Could you check a few things on this drawing? It's one solid part, dimensions in mm from its lowest x, y, z. Coordinates: 2 decimals unless noted, no trailing zeros. Order: outer loops, then holes, each group sorted by start corner. A loop starts at its lowest first (then second) coordinate and runs counter-clockwise, first axis right, second up. Notation, with made-up numbers: (31.25, 37.25) - (73.25, 37.25) arc R19 ccw to (73.25, 60.25) - close; hole circle Ø2 at (62, 21.25). An arc over 180 degrees is marked (long way). Answer in a Markdown table with one row per item. Add a question column.
Item 1: I want a section at C-C (x = 7.5). Please give me the cut outline in (y, z).
Item 2: I want a section at B-B (y = 7.5). Please give me the cut outline in (x, z), plus the area to 3 significant figures.
Item 3: If I drill on line 1 along Y through (x, z) = (7.5, 13.25); line 2 along X through (y, z) = (5.5, 34); line 3 along X through (y, z) = (5.25, 20), over which ranges is the centre line in solid material (lowest first)? Write a range as from..to.
Item 4: I want a section at A-A (z = 4). Please give me the cut outline in (x, y).
Item 5: Thinking about a two-plate mould opening in Y: for the marked faces 1 and 2, which applies, +Y half, -Y half, draft (parallel to the pull), parting line (faces both ways), or undercut?
Item 6: Will these pins go through, and if not, where does the flat tip stop? pin 1 Ø5 at (y, z) = (4.5, 30.5) entering from +X; pin 2 Ø4 at (x, z) = (13, 15.5) entering from +Y; pin 3 Ø2.5 at (y, z) = (6.5, 4.5) entering from +X; pin 4 Ø2 at (x, y) = (4.5, 5.5) entering from -Z.
Item 7: I want a section at D-D (z = 27.5). Please give me the cut outline in (x, y), plus the area to 3 significant figures.
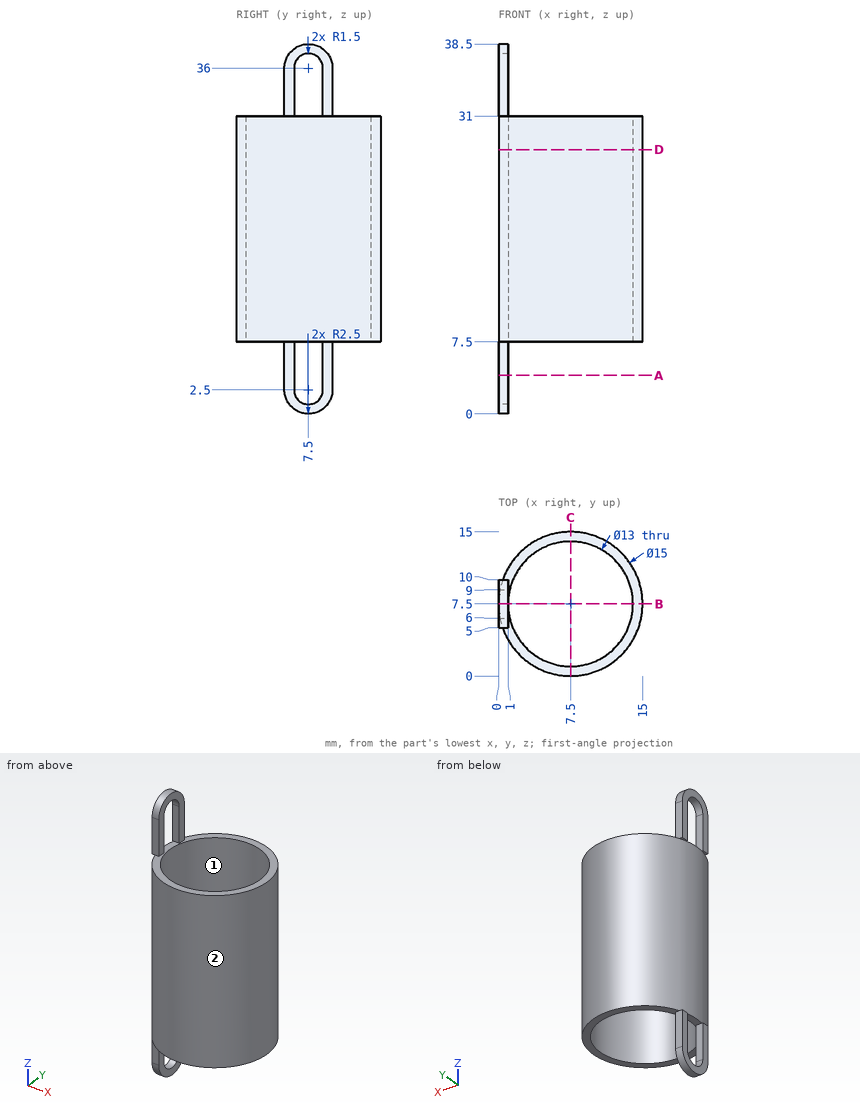
Values follow:
| question | item | result |
|---|---|---|
| 1 | outline | (0, 7.5) - (1, 7.5) - (1, 31) - (0, 31) - close; (14, 7.5) - (15, 7.5) - (15, 31) - (14, 31) - close |
| 2 | outline | (0, 0) - (1, 0) - (1, 1) - (0, 1) - close; (0, 7.5) - (1, 7.5) - (1, 31) - (0, 31) - close; (0, 37.5) - (1, 37.5) - (1, 38.5) - (0, 38.5) - close; (14, 7.5) - (15, 7.5) - (15, 31) - (14, 31) - close |
| 2 | area | 49.0 mm^2 |
| 3 | line 1 | y = 0..1, 14..15 |
| 3 | line 2 | x = 0..1 |
| 3 | line 3 | x = 0.35..1.4, 13.6..14.65 |
| 4 | outline | (0, 5) - (1, 5) - (1, 6) - (0, 6) - close; (0, 9) - (1, 9) - (1, 10) - (0, 10) - close |
| 5 | face 1 | undercut |
| 5 | face 2 | parting line |
| 6 | pin 1 | stops at x = 14.98 |
| 6 | pin 2 | stops at y = 14.13 |
| 6 | pin 3 | stops at x = 1 |
| 6 | pin 4 | passes through |
| 7 | outline | circle Ø15 at (7.5, 7.5); hole circle Ø13 at (7.5, 7.5) |
| 7 | area | 44.0 mm^2 |
